from build123d import *

# Parameters (mm, degrees)
SKETCH1_W           = 99
SKETCH1_H           = 62.5
BOSS_EXTRUDE1_DEPTH = 53.7
SKETCH2_W           = 79
SKETCH2_H           = 62.5
CUT_EXTRUDE1_DEPTH  = 50.7
SKETCH3_W           = 25
SKETCH3_H           = 62.5
BOSS_EXTRUDE2_DEPTH = 10
BOSS_EXTRUDE4_DEPTH = 3
SKETCH5_W           = 24
SKETCH5_H           = 62.5
CUT_EXTRUDE3_DEPTH  = 72
CUT_EXTRUDE4_REACH  = 96.863
SKETCH6_R           = 1
SKETCH7_R           = 2.5
CUT_EXTRUDE5_DEPTH  = 72


with BuildPart() as part:
    # Sketch1 → Boss-Extrude1 (new body)
    with BuildSketch(Plane(origin=(0, 0, 0), x_dir=(1, 0, 0), z_dir=(0, 1, 0))):
        with Locations((49.5, 31.25)):
            Rectangle(SKETCH1_W, SKETCH1_H)
    extrude(amount=BOSS_EXTRUDE1_DEPTH)

    # Sketch2 → Cut-Extrude1 (cut)
    with BuildSketch(Plane(origin=(0, 53.7, 0), x_dir=(1, 0, 0), z_dir=(0, 1, 0))):
        with Locations((49.5, 31.25)):
            Rectangle(SKETCH2_W, SKETCH2_H)
    extrude(amount=-CUT_EXTRUDE1_DEPTH, mode=Mode.SUBTRACT)

    # Sketch3 → Boss-Extrude2 (add)
    with BuildSketch(Plane(origin=(0, 3, 0), x_dir=(1, 0, 0), z_dir=(0, 1, 0))):
        with Locations((64.5, 31.25)):
            Rectangle(SKETCH3_W, SKETCH3_H)
    extrude(amount=BOSS_EXTRUDE2_DEPTH)

    # Sketch4 → Boss-Extrude4 (add)
    with BuildSketch(Plane.ZY.offset(-52)):
        Polygon((-62.5, 13), (-62.5, 39), (-52.5, 39), (-52.5, 18), (-10, 18), (-10, 39), (0, 39), (0, 13), align=None)
    extrude(amount=-BOSS_EXTRUDE4_DEPTH)

    # Sketch5 → Cut-Extrude3 (cut)
    with BuildSketch(Plane.XZ):
        with Locations((12, -31.25)):
            Rectangle(SKETCH5_W, SKETCH5_H)
    extrude(amount=-CUT_EXTRUDE3_DEPTH, mode=Mode.SUBTRACT)

    # Sketch6 → Cut-Extrude4 (cut, up to next)
    with BuildSketch(Plane.ZY.offset(-52), mode=Mode.PRIVATE) as cut_extrude4_sk1:
        with Locations((-56.25, 32)):
            Circle(SKETCH6_R)
    cut_extrude4_tool1 = extrude(cut_extrude4_sk1.sketch, amount=-CUT_EXTRUDE4_REACH, mode=Mode.PRIVATE) & part.part
    # Sketch6 → Cut-Extrude4 (cut, up to next)
    with BuildSketch(Plane.ZY.offset(-52), mode=Mode.PRIVATE) as cut_extrude4_sk2:
        with Locations((-56.25, 22)):
            Circle(SKETCH6_R)
    cut_extrude4_tool2 = extrude(cut_extrude4_sk2.sketch, amount=-CUT_EXTRUDE4_REACH, mode=Mode.PRIVATE) & part.part
    # Sketch6 → Cut-Extrude4 (cut, up to next)
    with BuildSketch(Plane.ZY.offset(-52), mode=Mode.PRIVATE) as cut_extrude4_sk3:
        with Locations((-6.25, 22)):
            Circle(SKETCH6_R)
    cut_extrude4_tool3 = extrude(cut_extrude4_sk3.sketch, amount=-CUT_EXTRUDE4_REACH, mode=Mode.PRIVATE) & part.part
    # Sketch6 → Cut-Extrude4 (cut, up to next)
    with BuildSketch(Plane.ZY.offset(-52), mode=Mode.PRIVATE) as cut_extrude4_sk4:
        with Locations((-6.25, 32)):
            Circle(SKETCH6_R)
    cut_extrude4_tool4 = extrude(cut_extrude4_sk4.sketch, amount=-CUT_EXTRUDE4_REACH, mode=Mode.PRIVATE) & part.part
    add(cut_extrude4_tool1.solids().sort_by_distance((52, 32, -56.25))[0], mode=Mode.SUBTRACT)
    add(cut_extrude4_tool2.solids().sort_by_distance((52, 22, -56.25))[0], mode=Mode.SUBTRACT)
    add(cut_extrude4_tool3.solids().sort_by_distance((52, 22, -6.25))[0], mode=Mode.SUBTRACT)
    add(cut_extrude4_tool4.solids().sort_by_distance((52, 32, -6.25))[0], mode=Mode.SUBTRACT)

    # Sketch7 → Cut-Extrude5 (cut)
    with BuildSketch(Plane(origin=(99, 0, 0), x_dir=(0, 0, -1), z_dir=(1, 0, 0))):
        with Locations((40.5, 28)):
            Circle(SKETCH7_R)
    extrude(amount=-CUT_EXTRUDE5_DEPTH, mode=Mode.SUBTRACT)


solid = part.part
Can you work these out from the model? Positions are in its coordinate system, mm. A direction names the side the tool comes from. Coordinates: 2 decimals unless noted, no trailing zeros. Order: outer loops, then holes, each group sorted by start corner. A loop starts at its lowest first (then second) coordinate and runs counter-clockwise, first axis right, second up. Notation, with made-up numbers: (7, 66.25) - (53, 66.25) arc R25 cw to (53, 97.25) - close; hole circle Ø5 at (-8, 87). An arc over 180 degrees is marked (long way). Answer as a JSON object with one key per item and string values. Group by question number.
Q1. Imagine slicing it at A-A (y = 28). Please give me the cut outline in (x, z), and give its area (3 significant figures).
Q2. On a 3-axis mill with a long thin cutter (end or side, diameter ignored), from which of +Z, -Z, +X, -X, +Y, -Y can I reach the whole of each face in a straight line? I mean faces 5 (the face through (53.479, 21.024, -6.467)), 6 (the face through (38, 3, -32)), 7 (the face through (53, 29, -52.5)). Say none if no direction works.
Q3. I need wall thicknesses on line 1 (Y direction, x = 54.05, z = -6.25); line 2 (X direction, y = 19, z = -58.5); line 3 (X direction, y = 12.5, z = -6.5). Which ranges of each line are inside material? Lowest first, please. Write a range as from..to.
Q4. We'd pull the mould along X, two halves only. Please class faces 1 (the face through (52, 17, -31)), 2 (the face through (66, 13, -32)), 3 (the face through (77, 8, -31)), 4 (the face through (53, 39, -5)): +X half, -X half, draft (parallel to the pull), parting line (faces both ways), or undercut.
Q5. Will these pins go through, and if not, where does the flat tip stop? P1, Ø8, axis at y = 8.5, z = -55, coming from the -X side; P2, Ø3.5, axis at x = 54, z = -2.5, coming from the +Y side; P3, Ø8, axis at x = 65.5, z = -54, coming from the +Y side.
Q6. Imagine slicing it at B-B (z = -42). Please give me the cut outline in (x, y).
Q7. Imagine slicing it at C-C (y = 22). Please give me the cut outline in (x, z), and give its area (3 significant figures).
Q8. Imagine slicing it at D-D (z = -56.25). Please give me the cut outline in (x, y), and give its area (3 significant figures).
Determined:
{
 "1": {"outline": "(52, -62.5) - (55, -62.5) - (55, -52.5) - (52, -52.5) - close; (52, -10) - (55, -10) - (55, 0) - (52, 0) - close; (89, -62.5) - (99, -62.5) - (99, -43) - (89, -43) - close; (89, -38) - (99, -38) - (99, 0) - (89, 0) - close", "area": "635 mm2"},
 "2": {"face 5": "-X", "face 6": "+Z, -Z, -X, +Y", "face 7": "-X, +Y"},
 "3": {"line 1": "y = 0..21, 23..31, 33..39", "line 2": "x = 52..55, 89..99", "line 3": "x = 52..77, 89..99"},
 "4": {"face 1": "-X half", "face 2": "undercut", "face 3": "undercut", "face 4": "draft"},
 "5": {"P1": "stops at x = 52", "P2": "stops at y = 39", "P3": "stops at y = 13"},
 "6": {"outline": "(24, 0) - (99, 0) - (99, 26) - (89, 26) - (89, 3) - (77, 3) - (77, 13) - (55, 13) - (55, 18) - (52, 18) - (52, 3) - (24, 3) - close; (89, 30) - (99, 30) - (99, 53.7) - (89, 53.7) - close"},
 "7": {"outline": "(52, -62.5) - (55, -62.5) - (55, -57.25) - (52, -57.25) - close; (52, -55.25) - (55, -55.25) - (55, -52.5) - (52, -52.5) - close; (52, -10) - (55, -10) - (55, -7.25) - (52, -7.25) - close; (52, -5.25) - (55, -5.25) - (55, 0) - (52, 0) - close; (89, -62.5) - (99, -62.5) - (99, 0) - (89, 0) - close", "area": "673 mm2"},
 "8": {"outline": "(24, 0) - (99, 0) - (99, 53.7) - (89, 53.7) - (89, 3) - (77, 3) - (77, 13) - (55, 13) - (55, 21) - (52, 21) - (52, 3) - (24, 3) - close; (52, 23) - (55, 23) - (55, 31) - (52, 31) - close; (52, 33) - (55, 33) - (55, 39) - (52, 39) - close", "area": "1,050 mm2"}
}
